from build123d import *

# Parameters (mm, degrees)
SKETCH1_R           = 25.5
BOSS_EXTRUDE1_DEPTH = 255
SKETCH5_R           = 15.5
BOSS_EXTRUDE2_DEPTH = 25


with BuildPart() as part:
    # Sketch1 → Boss-Extrude1 (new body)
    with BuildSketch(Plane(origin=(0, 0, 0), x_dir=(1, 0, 0), z_dir=(0, 1, 0))):
        with Locations(Location((0, 0, 0), (0, 0, 270))):
            Circle(SKETCH1_R)
    extrude(amount=BOSS_EXTRUDE1_DEPTH)

    # Sweep1: sweep along a path in Sketch4
    with BuildLine(Plane(origin=(0, 0, 0), x_dir=(0, 0, -1), z_dir=(1, 0, 0))) as sweep1_path:
        ThreePointArc((-200, 189.54), (-101.226787493, 219.07574986), (0, 199.54))
    # Sketch3 → Sweep1 (sweep)
    with BuildSketch(Plane.XY.offset(200)):
        with BuildLine():
            Line((-13.819688726, 197.030082188), (13.819688726, 197.030082188))
            ThreePointArc((13.819688726, 197.030082188), (21.309770914, 189.54), (13.819688726, 182.049917812))
            Line((13.819688726, 182.049917812), (-13.819688726, 182.049917812))
            ThreePointArc((-13.819688726, 182.049917812), (-21.309770914, 189.54), (-13.819688726, 197.030082188))
        make_face()
    sweep(path=sweep1_path.line)

    # Sketch5 → Boss-Extrude2 (add)
    with BuildSketch(Plane(origin=(0, 255, 0), x_dir=(1, 0, 0), z_dir=(0, 1, 0))):
        with Locations(Location((0, 0, 0), (0, 0, 270))):
            Circle(SKETCH5_R)
    extrude(amount=BOSS_EXTRUDE2_DEPTH)


solid = part.part
CAD build for the part. Positions are in the model's coordinates, mm. A direction names the side the tool comes from. Round coordinates to 2 decimals unless told otherwise and drop trailing zeros. Order: outer loops, then holes, each group sorted by start corner. A loop starts at its lowest first (then second) coordinate and runs counter-clockwise, first axis right, second up. Notation, with made-up numbers: (-7, 79) -> (15, 79) arc R20 cw to (15, 84) -> close; hole circle Ø9 at (64.5, 34.25). An arc over 180 degrees is marked (long way). Write item = value, one per line. Start each with the question number.
(1) Cut at B-B, the plane x = 0. List the corners of the cut face in (y, z), then the cut area to 3 significant figures.
(2) Cut at A-A, the plane z = 0. List the corners of the cut face in (x, y).
(3) Pull direction Z, two halves, no side cores. Call faces 3 (the flat face through (0, 190, 200)), 4 (the flat face through (0, 0, 0)), 5 (the cylindrical face through (-0.193, 224.598, 113.878)): released by +Z, released by -Z, zero draft, split by the parting line, or undercut.
(4) Pin check, flat tips, straight feed: P1, Ø3, axis at y = 233, z = 7, coming from the -X side; P2, Ø10, axis at x = 10, z = 51.5, coming from the -Y side; P3, Ø8, axis at y = 141, z = 23, coming from the +X side. Stop position of each tip, or through.
(5) Cut at C-C, the plane y = 120. List the corners of the cut face in (x, z).
(6) Probe line 1 (Y direction, x = -6, z = 91); line 2 (Z direction, x = 17, y = 188); line 3 (Y direction, x = -16.5, z = 31.5). List the from-to ranges inside material, lowest first. Write a range as [from, to].
(7) Which spindle directions (+Z, -Z, +X, -X, +Y, -Y) get a long thin tool onto all of the face, cutting with end or side? Do faces 1 (the flat face through (-17, 255, 0)), 2 (the flat face through (0, 280, 0)). Say none if no direction does.
Model answer:
q1.outline = (0, -25.5) -> (255, -25.5) -> (255, -15.5) -> (280, -15.5) -> (280, 15.5) -> (255, 15.5) -> (255, 25.5) -> (216.17, 25.5) arc R222.81 ccw to (197.03, 200) -> (182.05, 200) arc R209.9 cw to (202.63, 25.5) -> (0, 25.5) -> close
q1.area = 16,100 mm2
q2.outline = (-25.5, 0) -> (25.5, 0) -> (25.5, 255) -> (15.5, 255) -> (15.5, 280) -> (-15.5, 280) -> (-15.5, 255) -> (-25.5, 255) -> close
q3.face_3 = released by +Z
q3.face_4 = zero draft
q3.face_5 = undercut
q4.P1 = -24.9
q4.P2 = 208.27
q4.P3 = 17.01
q5.outline = circle Ø51 at (0, 0)
q6.line_1 = [212.92, 225.84]
q6.line_2 = [-19.01, 19.01], [190.9, 200]
q6.line_3 = [204.92, 217.46]
q7.face_1 = +Y
q7.face_2 = +Z, -Z, +X, -X, +Y
